For this review, take the finished solid that the model builds, in its own axes (mm). Face numbers are marked on the shaded views. Coordinates: 2 decimals unless noted, no trailing zeros. Order: outer loops, then holes, each group sorted by start corner. A loop starts at its lowest first (then second) coordinate and runs counter-clockwise, first axis right, second up. Notation, with made-up numbers: (16, -24.5) -> (75, -24.5) arc R28 ccw to (75, 7.5) -> close; hole circle Ø7 at (20.5, 45.25). An arc over 180 degrees is marked (long way). Write item = value, one per line. Start each with the question number.
1) Wall thickness on probe 1 along X at (y, z) = (34, 9.5); probe 2 along Y at (x, z) = (26.5, 18); probe 3 along X at (y, z) = (-18.5, 3.25): over which ranges is each line inside the solid? List them lowest first. Write a range as [from, to].
2) Insertion check: pin 1 Ø12 at (x, y) = (-17, -11.5) entering from -Z. The pin has a flat end and moves straight along its axis. Give the tip position at first contact, or say it passes through.
3) Consider section A-A on x = 0. State how many separate pieces and enclosed holes the cut face has, and give its area (3 significant figures).
4) Draft analysis for pull direction Y (two halves, no side actions). For the marked faces 1, 2 and 3, state which applies: +Y half, -Y half, draft (parallel to the pull), parting line (faces both ways), or undercut.
5) Consider section D-D on y = -38.1. Give the boundary of the cut face in (x, z) (3 decimals), and give its area (3 significant figures).
6) Consider section B-B on y = 0. Give the boundary of the cut face in (x, z), and give its area (3 significant figures).
from build123d import *

# Parameters (mm, degrees)
F0_W     = 76.2
F0_H     = 88.9
F0_R     = 3.175
F0_R_2   = 29.9085
F1_DEPTH = 19.05
F2_R     = 3.175
F3_DEPTH = 25.4
F4_R     = 3.175
F5_DEPTH = 25.4


with BuildPart() as f1:
    # F0 (on Top) → F1 (new body)
    with BuildSketch(Plane.XY):
        Rectangle(F0_W, F0_H)
        with Locations((0, -38.1)):
            Circle(F0_R, mode=Mode.SUBTRACT)
        Circle(F0_R_2, mode=Mode.SUBTRACT)
    extrude(amount=F1_DEPTH)

    # F2 (on face) → F3 (cut)
    with BuildSketch(Plane.YZ.offset(38.1)):
        with Locations((0, 9.525)):
            Circle(F2_R)
    extrude(amount=-F3_DEPTH, mode=Mode.SUBTRACT)

    # F4 (on face) → F5 (cut)
    with BuildSketch(Plane(origin=(0, 44.45, 0), x_dir=(-1, 0, 0), z_dir=(0, 1, 0))):
        with Locations((0, 9.525)):
            Circle(F4_R)
    extrude(amount=-F5_DEPTH, mode=Mode.SUBTRACT)


solid = f1.part
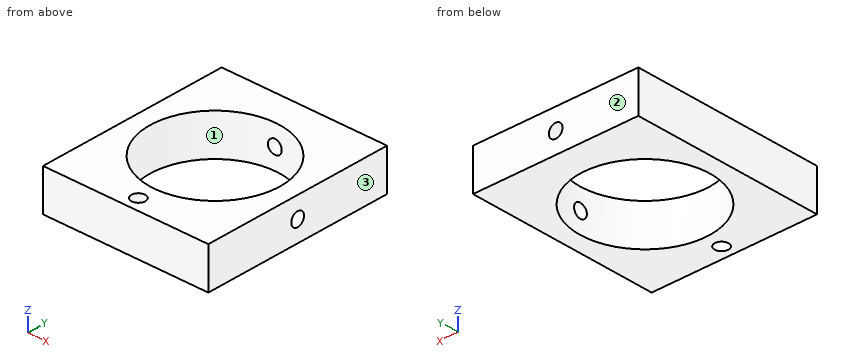
Answer sheet:
q1.probe_1 = [-38.1, -3.17], [3.17, 38.1]
q1.probe_2 = [-44.45, -13.87], [13.87, 44.45]
q1.probe_3 = [-38.1, -23.5], [23.5, 38.1]
q2.pin_1 = through
q3.separate_pieces = 4
q3.enclosed_holes = 0
q3.area = 341 mm2
q4.face_1 = undercut
q4.face_2 = +Y half
q4.face_3 = draft
q5.outline = (-38.1, 0) -> (-3.175, 0) -> (-3.175, 19.05) -> (-38.1, 19.05) -> close; (3.175, 0) -> (38.1, 0) -> (38.1, 19.05) -> (3.175, 19.05) -> close
q5.area = 1,330 mm2
q6.outline = (-38.1, 0) -> (-29.91, 0) -> (-29.91, 19.05) -> (-38.1, 19.05) -> close; (29.91, 0) -> (38.1, 0) -> (38.1, 6.35) -> (29.91, 6.35) -> close; (29.91, 12.7) -> (38.1, 12.7) -> (38.1, 19.05) -> (29.91, 19.05) -> close
q6.area = 260 mm2
